Verification items for the finished model (mm, model axes). Face numbers are marked on the shaded views. A direction names the side the tool comes from. Coordinates: 2 decimals unless noted, no trailing zeros. Write each loop counter-clockwise with the first axis right and the second up, starting at its lowest first coordinate (ties: lowest second). Pieces come first, ordered by that corner, then holes. Notation, with made-up numbers: M 44.5,-11.5 L 86.5,-11.5 A29 cw 86.5,15.5 Z; hole C -4,8 d7. An arc over 180 degrees is marked long. One line per item, written item: value.
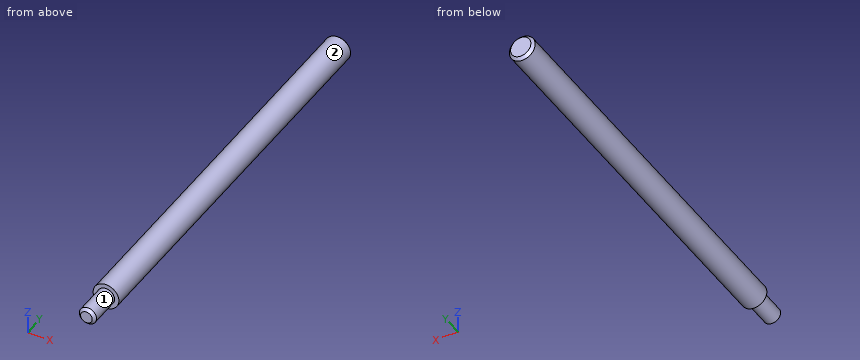
```python
from build123d import *

# Parameters (mm, degrees)
F0_R     = 2.3876
F1_DEPTH = 75.565
F2_R     = 1.5875
F3_DEPTH = 6.35
F4_SIZE  = 0.508


with BuildPart() as f1:
    # F0 (on Front) → F1 (new body)
    with BuildSketch(Plane.XZ):
        Circle(F0_R)
    extrude(amount=F1_DEPTH)

    # F2 (on face) → F3 (join)
    with BuildSketch(Plane.XZ.offset(75.565)):
        Circle(F2_R)
    extrude(amount=F3_DEPTH)

    # F4
    f4_edges = [f1.edges().sort_by_distance(p)[0] for p in [
        (-1.5875, -81.915, 0),
        (-2.3876, 0, 0),
    ]]
    chamfer(f4_edges, length=F4_SIZE)


solid = f1.part
```
Item 1: Scan lines: line 1 (Z direction, x = 0.2, y = -57); line 2 (Y direction, x = 0.7, z = -1.65) (3 decimals); line 3 (X direction, y = -8, z = -0.5). Record each from-to range of solid material in increasing order.
The answers:
line 1: z = -2.38 to 2.38
line 2: y = -75.565 to 0
line 3: x = -2.33 to 2.33
Item 2: Access from +Z, -Z, +X, -X, +Y, -Y to the whole of each face (thin tool, end or side, straight path). Record for the marked faces 1 and 2.
The answers:
face 1: -Y
face 2: +Y, -Y
Item 3: Go/stop test with a flat-tipped pin: P1, Ø1, axis at y = -63.5, z = -1.5, coming from the +X side. Record where the tip stops, or that it passes through.
The answers:
P1: stops at x = 2.17
Item 4: Cross-section at A-A, the plane z = 0. Enter the section's corners in (x, y) (1 decimal), and give its area (3 significant figures).
The answers:
outline: M -2.4,-75.6 L -1.6,-75.6 L -1.6,-81.4 L -1.1,-81.9 L 1.1,-81.9 L 1.6,-81.4 L 1.6,-75.6 L 2.4,-75.6 L 2.4,-0.5 L 1.9,0 L -1.9,0 L -2.4,-0.5 Z
area: 380 mm²
Item 5: Cross-section at C-C, the plane y = -4.5. Enter the section's corners in (x, z).
The answers:
outline: C 0,0 d4.78
Item 6: Cross-section at B-B, the plane x = 0. Enter the section's corners in (y, z) (1 decimal).
The answers:
outline: M -81.9,-1.1 L -81.4,-1.6 L -75.6,-1.6 L -75.6,-2.4 L -0.5,-2.4 L 0,-1.9 L 0,1.9 L -0.5,2.4 L -75.6,2.4 L -75.6,1.6 L -81.4,1.6 L -81.9,1.1 Z
